Autodesk Fusion 360 part; units mm, degrees
sketch "Esquisse1" plane through (0, 0, 0) normal (0, 0, 1) x (1, 0, 0)
  line L0 (-12.5, 12.5) -> (12.5, 12.5)
  line L1 (12.5, 12.5) -> (12.5, -12.5)
  line L2 (12.5, -12.5) -> (-12.5, -12.5)
  line L3 (-12.5, -12.5) -> (-12.5, 12.5)
  circle A0 centre (-10.5, 10.5) radius 1
  circle A1 centre (10.5, 10.5) radius 1
  circle A2 centre (-10.5, -2) radius 1
  circle A3 centre (10.5, -2) radius 1
  dimension "d1" = 25
  dimension "d2" = 25
  dimension "d3" = 12.5
  dimension "d4" = 12.5
  dimension "d5" = 21
  dimension "d6" = 2
  dimension "d7" = 2
  dimension "d8" = 2
  dimension "d9" = 2
  dimension "d10" = 2
  dimension "d11" = 12.5
  dimension "d12" = 12.5
  dimension "d13" = 21
  dimension "d14" = 2
  dimension "d15" = 2
  dimension "d16" = 2
  dimension "d17" = 2
extrude "Extrusion1" add sketch "Esquisse1" along normal blind 1
sketch "Esquisse2" plane through (0, 0, 0) normal (0, 0, -1) x (1, 0, 0)
  circle A0 centre (-10.5, 2) radius 1
  circle A1 centre (10.5, -10.5) radius 1
  circle A2 centre (10.5, 2) radius 1
  circle A3 centre (-10.5, -10.5) radius 1
  line L0 (12.5, 12.5) -> (-12.5, 12.5)
  line L1 (-12.5, 12.5) -> (-12.5, -12.5)
  line L2 (-12.5, -12.5) -> (12.5, -12.5)
  line L3 (12.5, -12.5) -> (12.5, 12.5)
  circle A4 centre (-10.5, -10.5) radius 2
  circle A5 centre (-10.5, 2) radius 2
  circle A6 centre (10.5, 2) radius 2
  circle A7 centre (10.5, -10.5) radius 2
  circle A8 centre (-10.5, 2) radius 1
  circle A9 centre (10.5, 2) radius 1
  circle A10 centre (-10.5, -10.5) radius 1
  circle A11 centre (10.5, -10.5) radius 1
  dimension "d20" = 4
  dimension "d21" = 4
  dimension "d22" = 4
  dimension "d23" = 4
  dimension "d26" = 2
extrude "Extrusion2" add sketch "Esquisse2" along normal blind 3 contours A5 | A6 | A7 | A4
sketch "Esquisse3" plane through (0, 0, 1) normal (0, 0, 1) x (-1, 0, 0)
  circle A0 centre (10.5, 2) radius 1
  circle A1 centre (-10.5, 2) radius 1
  circle A2 centre (-10.5, -10.5) radius 1
  circle A3 centre (10.5, -10.5) radius 1
  line L0 (12.5, 12.5) -> (-12.5, 12.5)
  line L1 (-12.5, 12.5) -> (-12.5, -12.5)
  line L2 (-12.5, -12.5) -> (12.5, -12.5)
  line L3 (12.5, -12.5) -> (12.5, 12.5)
  circle A4 centre (10.5, -10.5) radius 1.6
  circle A5 centre (-10.5, -10.5) radius 1.6
  circle A6 centre (-10.5, 2) radius 1.6
  circle A7 centre (10.5, 2) radius 1.6
  dimension "d27" = 3.2
  dimension "d28" = 3.2
  dimension "d29" = 3.2
  dimension "d30" = 3.2
extrude "Extrusion3" cut sketch "Esquisse3" against normal blind 0.5 contours A4 | A5 | A6 | A7
Read the model definition and answer for the solid it produces. Units are mm, in the model's axes. A direction names the side the tool comes from. Round coordinates to 2 decimals unless told otherwise and drop trailing zeros. Write each loop counter-clockwise with the first axis right and the second up, starting at its lowest first coordinate (ties: lowest second). Pieces come first, ordered by that corner, then holes. Notation, with made-up numbers: M 44.25,-5 L 59.25,-5 A25 cw 59.25,10 Z; hole C -20.5,52.25 d5. An arc over 180 degrees is marked long. Use a Markdown table: item, result.
1) Flat-ended cylindrical pins translate along their axes: pin 1 (2.5 mm diameter, centred on x = -10.5, y = 10.5, fed in from +Z); pin 2 (1 mm diameter, centred on x = -3.5, y = 3.5, fed in from -Z). Find the tip coordinate at first contact, or state that the pin passes through.
Answers follow:
| item | result |
|---|---|
| pin 1 | stops at z = 0.5 |
| pin 2 | stops at z = 0 |
2) Straight lines are drawn through the part: line 1 along X through (y, z) = (-2, -0.85); line 2 along Y through (x, z) = (-10.5, 0.7); line 3 along X through (y, z) = (-2, 0.6). For each, find the intervals that lie inside material, in ascending order. Write a range as [from, to].
Answers follow:
| item | result |
|---|---|
| line 1 | x = [-12.5, -11.5], [-9.5, -8.5], [8.5, 9.5], [11.5, 12.5] |
| line 2 | y = [-12.5, -3.6], [-0.4, 8.9], [12.1, 12.5] |
| line 3 | x = [-12.5, -12.1], [-8.9, 8.9], [12.1, 12.5] |
3) The part is cut by section A-A (z = -0.8). Write down the section's boundary in (x, y), plus the area to 3 significant figures.
Answers follow:
| item | result |
|---|---|
| outline | C -10.5,-2 d4; C -10.5,10.5 d4; C 10.5,-2 d4; C 10.5,10.5 d4; hole C -10.5,-2 d2; hole C -10.5,10.5 d2; hole C 10.5,-2 d2; hole C 10.5,10.5 d2 |
| area | 37.7 mm2 |
4) The part is cut by section B-B (x = 7). Write down the section's boundary in (y, z), plus the area to 3 significant figures.
Answers follow:
| item | result |
|---|---|
| outline | M -12.5,0 L 12.5,0 L 12.5,1 L -12.5,1 Z |
| area | 25.0 mm2 |
5) For a pull along Y with two mould halves and no side action, classify faces 1 (the flat face through (-12.1, 12, 0)), 2 (the cylindrical face through (11.77, 11.47, 0.75)) as pulls with the +Y half, pulls with the -Y half, needs draft (parallel to the pull), parting line crosses it, or undercut.
Answers follow:
| item | result |
|---|---|
| face 1 | needs draft |
| face 2 | undercut |
6) A tool of negligible diameter and unlimited length cuts with its end or side. For faces 3 (the flat face through (0, 0, 1)), 4 (the flat face through (12, 12.1, 0)), 5 (the cylindrical face through (-10.63, 9.51, -1.27)), 6 (the cylindrical face through (-10.76, 12.483, -1.479)), 7 (the cylindrical face through (-9.23, 11.47, 0.75)), from which of +Z, -Z, +X, -X, +Y, -Y can it reach the whole face along a straight path? Write none if from no direction.
Answers follow:
| item | result |
|---|---|
| face 3 | +Z, +X, -X, +Y, -Y |
| face 4 | -Z, +X, +Y |
| face 5 | +Z, -Z |
| face 6 | -Z |
| face 7 | +Z |
